For this review, use the dimensioned drawing (mm, ordinates from the lowest corner) and the shaded views. A direction names the side the tool comes from. Coordinates: 2 decimals unless noted, no trailing zeros. Write each loop counter-clockwise with the first axis right and the second up, starting at its lowest first coordinate (ties: lowest second). Pieces come first, ordered by that corner, then holes.
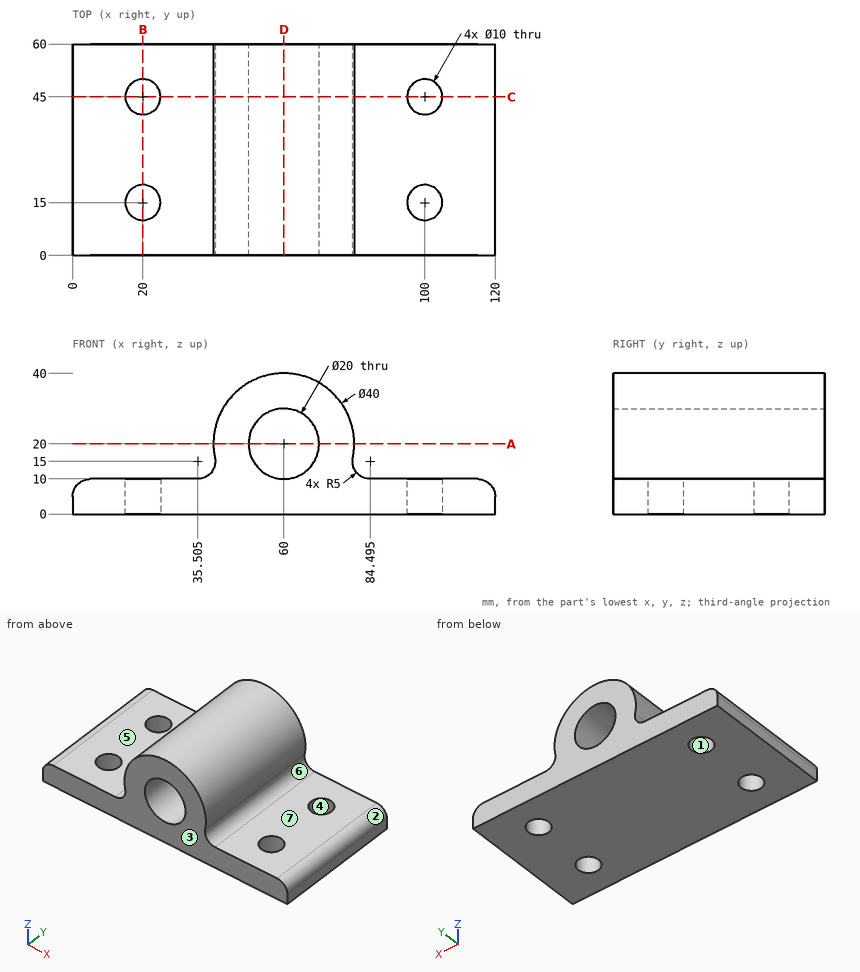
(1) Wall thickness on line 1 (Y direction, x = 100, z = 6.75); line 2 (Z direction, x = 59.5, y = 10.5); line 3 (Z direction, x = 33.5, y = 57.5): over which ranges is each line inside the solid? List them lowest first.
(2) Consider section B-B (x = 20). Give the boundary of the cut face in (y, z).
(3) For the marked faces 5, 6 and 7, list the 3-axis set-ups (+Z, -Z, +X, -X, +Y, -Y) from which the entire face can be reached by the end or side of a thin tool; tool diameter is ignored.
(4) Consider section D-D (x = 60). Give the boundary of the cut face in (y, z), plus the area to 3 significant figures.
(5) Mouldability with a two-part tool opening along Y and no side actions: class the marked faces 1, 2, 3 and 4 as +Y half, -Y half, draft (parallel to the pull), parting line (faces both ways), or undercut.
(6) Insertion check: pin 1 Ø4 at (x, y) = (97.5, 26.5) entering from +Z; pin 2 Ø2 at (y, z) = (17, 10.5) entering from -X; pin 3 Ø1 at (y, z) = (11.5, 33.5) entering from -X. Each pin has a flat end and moves straight along its axis. Give the tip position at first contact, or say it passes through.
(7) Consider section A-A (z = 20). Give the boundary of the cut face in (x, y).
(8) Consider section C-C (y = 45). Give the boundary of the cut face in (x, z) (3 decimals).
Results:
1. line 1: y = 0 to 10, 20 to 40, 50 to 60
1. line 2: z = 0 to 10.01, 29.99 to 39.99
1. line 3: z = 0 to 10
2. outline: (0, 0) - (10, 0) - (10, 10) - (0, 10) - close; (20, 0) - (40, 0) - (40, 10) - (20, 10) - close; (50, 0) - (60, 0) - (60, 10) - (50, 10) - close
3. face 5: +Z, -X, +Y, -Y
3. face 6: +X, +Y, -Y
3. face 7: +Z, +X, +Y, -Y
4. outline: (0, 0) - (60, 0) - (60, 10) - (0, 10) - close; (0, 30) - (60, 30) - (60, 40) - (0, 40) - close
4. area: 1,200 mm2
5. face 1: undercut
5. face 2: draft
5. face 3: -Y half
5. face 4: undercut
6. pin 1: stops at z = 10
6. pin 2: stops at x = 2.82
6. pin 3: stops at x = 44.8
7. outline: (40, 0) - (50, 0) - (50, 60) - (40, 60) - close; (70, 0) - (80, 0) - (80, 60) - (70, 60) - close
8. outline: (0, 0) - (15, 0) - (15, 10) - (5, 10) arc R5 ccw to (0, 5) - close; (25, 0) - (95, 0) - (95, 10) - (84.495, 10) arc R5 cw to (79.596, 16) arc R20 ccw (long way) to (40.404, 16) arc R5 cw to (35.505, 10) - (25, 10) - close; (105, 0) - (120, 0) - (120, 5) arc R5 ccw to (115, 10) - (105, 10) - close; hole circle Ø20 at (60, 20)
